Build history of the part. All positions in model axes, mm. A direction names the side the tool comes from. Give positions to 0.01 mm unless a question says otherwise; leave off trailing zeros. Order: outer loops, then holes, each group sorted by start corner. A loop starts at its lowest first (then second) coordinate and runs counter-clockwise, first axis right, second up. Notation, with made-up numbers: (-36, 24.25) - (0, 24.25) arc R15 ccw to (0, 33.25) - close; hole circle Ø7 at (51.25, 71.5). An arc over 180 degrees is marked (long way). Use a Markdown table: item, result. Add a question column.
(1) Which spindle directions (+Z, -Z, +X, -X, +Y, -Y) get a long thin tool onto all of the face, cutting with end or side? Do faces 1 (the face through (-40, 60, 1)), 2 (the face through (-1, 39, -50)), 3 (the face through (25, 63, 0)). Say none if no direction does.
(2) Mould opens along Z. For faces 4 (the face through (-1, 39, 50)), 5 (the face through (-75, 39, 1)), 6 (the face through (50.35, 57.815, -12.675)) say: +Z half, -Z half, draft (parallel to the pull), parting line (faces both ways), or undercut.
(3) Slice it at D-D (y = 50). Write the cut outline in (x, z), then the cut area to 3 significant figures.
(4) Slice it at B-B (z = -23). Write the cut outline in (x, y).
(5) Flat gauge pins, fed straight in: pin 1 (16 mm diameter, centred on x = -23, z = -25, fed in from +Y); pin 2 (10 mm diameter, centred on y = 71, z = 13.5, fed in from +X). Where does each tip first touch, or does it go through?
(6) Slice it at A-A (y = 62). Write the cut outline in (x, z).
(7) Slice it at C-C (x = 48). Write the cut outline in (y, z), then the cut area to 4 significant figures.
(8) Wall check: line 1 (X direction, y = 55, z = -5.5); line 2 (X direction, y = 61, z = -20); line 3 (Y direction, x = -36, z = 41). Give the ranges that are in metal, low to high.
from build123d import *

# Parameters (mm, degrees)
SKETCH1_W               = 150
SKETCH1_H               = 100
BOSS_EXTRUDE1_DEPTH     = 80
CUT_EXTRUDE1_DEPTH      = 50
CUT_EXTRUDE2_DEPTH      = 1
CUT_EXTRUDE2_DEPTH_BACK = 101


with BuildPart() as part:
    # Sketch1 → Boss-Extrude1 (new body)
    with BuildSketch(Plane(origin=(0, 0, 0), x_dir=(1, 0, 0), z_dir=(0, 1, 0))):
        Rectangle(SKETCH1_W, SKETCH1_H)
    extrude(amount=BOSS_EXTRUDE1_DEPTH)

    # Sketch2 → Cut-Extrude1 (cut)
    with BuildSketch(Plane(origin=(75, 0, 0), x_dir=(0, 0, -1), z_dir=(1, 0, 0))):
        Polygon((-25, 80), (25, 80), (0, 35), align=None)
    extrude(amount=-CUT_EXTRUDE1_DEPTH, mode=Mode.SUBTRACT)

    # Sketch3 → Cut-Extrude2 (cut, two sides)
    with BuildSketch(Plane.XY.offset(50)) as cut_extrude2_sk:
        Polygon((-425, 80), (-75, 80), (-50, 80), (-50, 60), (-30, 60), (-30, 40), (-10, 40), (-10, 60), (10, 60), (10, 80), (10, 430), (-428.813790469, 975.382853869), (-863.813790469, 625.382853869), align=None)
    extrude(amount=CUT_EXTRUDE2_DEPTH, mode=Mode.SUBTRACT)
    extrude(cut_extrude2_sk.sketch, amount=-CUT_EXTRUDE2_DEPTH_BACK, mode=Mode.SUBTRACT)


solid = part.part
Solution:
| question | item | result |
|---|---|---|
| 1 | face 1 | +Z, -Z, +Y |
| 1 | face 2 | -Z, +X, -X, +Y, -Y |
| 1 | face 3 | +X, +Y |
| 2 | face 4 | +Z half |
| 2 | face 5 | draft |
| 2 | face 6 | undercut |
| 3 | outline | (-75, -50) - (-30, -50) - (-30, 50) - (-75, 50) - close; (-10, -50) - (75, -50) - (75, -8.33) - (25, -8.33) - (25, 8.33) - (75, 8.33) - (75, 50) - (-10, 50) - close |
| 3 | area | 12,200 mm2 |
| 4 | outline | (-75, 0) - (75, 0) - (75, 76.4) - (25, 76.4) - (25, 80) - (10, 80) - (10, 60) - (-10, 60) - (-10, 40) - (-30, 40) - (-30, 60) - (-50, 60) - (-50, 80) - (-75, 80) - close |
| 5 | pin 1 | y = 60 |
| 5 | pin 2 | x = 25 |
| 6 | outline | (-75, -50) - (-50, -50) - (-50, 50) - (-75, 50) - close; (10, -50) - (75, -50) - (75, -15) - (25, -15) - (25, 15) - (75, 15) - (75, 50) - (10, 50) - close |
| 7 | outline | (0, -50) - (80, -50) - (80, -25) - (35, 0) - (80, 25) - (80, 50) - (0, 50) - close |
| 7 | area | 6,875 mm2 |
| 8 | line 1 | -75 to -30, -10 to 25 |
| 8 | line 2 | -75 to -50, 10 to 75 |
| 8 | line 3 | 0 to 60 |
